Read the model definition and answer for the solid it produces. Units are mm, in the model's axes. A direction names the side the tool comes from. Coordinates: 2 decimals unless noted, no trailing zeros. Order: outer loops, then holes, each group sorted by start corner. A loop starts at its lowest first (then second) coordinate and runs counter-clockwise, first axis right, second up.
from build123d import *

# Parameters (mm, degrees)
SKETCH1_R             = 7.5
BOSS_EXTRUDE1_DEPTH   = 2
SKETCH2_R             = 9
BOSS_EXTRUDE2_DEPTH   = 0.9
SKETCH3_R             = 10
BOSS_EXTRUDE3_DEPTH   = 23
SKETCH5_R             = 2.1
CUT_EXTRUDE1_DEPTH    = 5.5
CUT_EXTRUDE2_DEPTH    = 20
SKETCH7_R             = 2.6
CUT_EXTRUDE3_DEPTH    = 30.509489999
CIRPATTERN1_OUTLINE_R = 2.6
CIRPATTERN1_DEPTH     = 10.0000001
CHAMFER1_SIZE         = 0.3


# Read off the part's stored shape, not the designer's step: CirPattern1
with BuildPart() as part:
    # Sketch1 → Boss-Extrude1 (new body)
    with BuildSketch(Plane(origin=(0, 0, 0), x_dir=(1, 0, 0), z_dir=(0, 1, 0))):
        with Locations(Location((0, 0, 0), (0, 0, 270))):
            Circle(SKETCH1_R)
    extrude(amount=BOSS_EXTRUDE1_DEPTH)

    # Sketch2 → Boss-Extrude2 (add)
    with BuildSketch(Plane(origin=(0, 2, 0), x_dir=(1, 0, 0), z_dir=(0, 1, 0))):
        with Locations(Location((0, 0, 0), (0, 0, 270))):
            Circle(SKETCH2_R)
    extrude(amount=BOSS_EXTRUDE2_DEPTH)

    # Sketch3 → Boss-Extrude3 (add)
    with BuildSketch(Plane(origin=(0, 2.9, 0), x_dir=(1, 0, 0), z_dir=(0, 1, 0))):
        with Locations(Location((0, 0, 0), (0, 0, 270))):
            Circle(SKETCH3_R)
    extrude(amount=BOSS_EXTRUDE3_DEPTH)

    # Sketch5 → Cut-Extrude1 (cut)
    with BuildSketch(Plane.XZ):
        with Locations(Location((4, 0, 0), (0, 0, 270))):
            Circle(SKETCH5_R)
        with Locations(Location((-2, -3.464101615, 0), (0, 0, 270))):
            Circle(SKETCH5_R)
        with Locations(Location((-2, 3.464101615, 0), (0, 0, 270))):
            Circle(SKETCH5_R)
    extrude(amount=-CUT_EXTRUDE1_DEPTH, mode=Mode.SUBTRACT)

    # Sketch6 → Cut-Extrude2 (cut)
    with BuildSketch(Plane(origin=(0, 25.9, 0), x_dir=(1, 0, 0), z_dir=(0, 1, 0))):
        with BuildLine():
            Line((-1.5, 2), (1.5, 2))
            ThreePointArc((1.5, 2), (0, -2.5), (-1.5, 2))
        make_face()
    extrude(amount=-CUT_EXTRUDE2_DEPTH, mode=Mode.SUBTRACT)

    # Sketch7 → Cut-Extrude3 (cut, through all)
    with BuildSketch(Plane.XY):
        with Locations(Location((0, 18.9, 0), (0, 0, 344.057631394))):
            Circle(SKETCH7_R)
    extrude(amount=-CUT_EXTRUDE3_DEPTH, mode=Mode.SUBTRACT)

    # CirPattern1 outline → CirPattern1 (cut)
    with BuildSketch(Plane(origin=(0, 0, 0), x_dir=(0.7071067811865509, 0, -0.707106781186544), z_dir=(0.707106781186544, 0, 0.707106781186551))):
        with Locations((0, 18.9)):
            Circle(CIRPATTERN1_OUTLINE_R)
    extrude(amount=CIRPATTERN1_DEPTH, mode=Mode.SUBTRACT)

    # Chamfer1
    chamfer1_edges = [part.edges().sort_by_distance(p)[0] for p in [
        (0, 0, -7.5),
    ]]
    chamfer(chamfer1_edges, length=CHAMFER1_SIZE)


solid = part.part
Q1. Determine the mould class of faces 1 (the cylindrical face through (-1.36, 21.116, -6.041)), 2 (the cylindrical face through (2.8, 17.3, 5.7)), 3 (the cylindrical face through (-4.05, 2.71, -3.01)), 4 (the flat face through (7.4, 2, -2)) for opening direction Y: +Y half, -Y half, draft (parallel to the pull), parting line (faces both ways), or undercut.
Q2. Which of the six approach directions +Z, -Z, +X, -X, +Y, -Y give full straight-line access (tool end or side, diameter ignored) to faces 5 (the flat face through (0, 0, 0)), 6 (the cylindrical face through (0.33, 1.138, -7.493)), 7 (the flat face through (0, 5.9, 0))?
Q3. The part is cut by section A-A, the plane y = 8. Determine the outline of the cut face in (x, z).
Q4. Each of these flat-tipped pins is pushed along its axis until it touches: P1, Ø6.5, axis at x = -2, z = 3.46, coming from the -Y side; P2, Ø2, axis at y = 4, z = -8, coming from the +X side; P3, Ø1.3, axis at x = -2.5, z = -4.5, coming from the -Y side; P4, Ø1.5, axis at y = 19.5, z = 1.5, coming from the +X side. Where does it stop, or does it pass through?
Q5. The part is cut by section B-B, the plane y = 2.5. Determine the outline of the cut face in (x, z).
Q6. Straight lines are drawn through the part: L1, parallel to X at y = 3.7, z = 0; L2, parallel to Y at x = 0, z = -4.5; L3, parallel to X at y = 13.25, z = 0. For each, find the intervals that lie inside material, in ascending order.
Computed values:
1. face 1: undercut
1. face 2: undercut
1. face 3: draft
1. face 4: -Y half
2. face 5: +Z, -Z, +X, -X, -Y
2. face 6: -Y
2. face 7: +Y
3. outline: circle Ø20 at (0, 0); hole (-1.5, -2) - (1.5, -2) arc R2.5 ccw (long way) to start
4. P1: stops at y = 0
4. P2: stops at x = 7.14
4. P3: stops at y = 5.5
4. P4: stops at x = 9.97
5. outline: circle Ø18 at (0, 0); hole circle Ø4.2 at (-2, -3.46); hole circle Ø4.2 at (-2, 3.46); hole circle Ø4.2 at (4, 0)
6. L1: x = -10 to 1.9, 6.1 to 10
6. L2: y = 0 to 16.3, 21.5 to 25.9
6. L3: x = -10 to -2.5, 2.5 to 10
